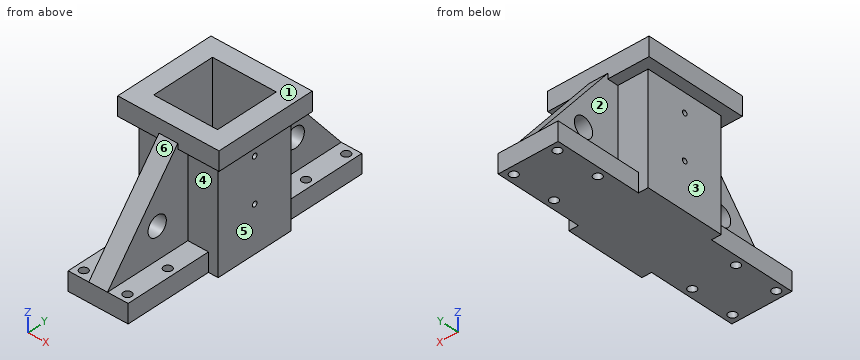
from build123d import *

# Parameters (mm, degrees)
SKETCH_W        = 48
SKETCH_H        = 15
PAD_DEPTH       = 203.2
SKETCH001_R     = 3.3
POCKET_DEPTH    = 15
SKETCH002_W     = 63.5
SKETCH002_H     = 63.5
PAD001_DEPTH    = 101.6
SKETCH003_W     = 51.05
SKETCH003_H     = 51.05
POCKET001_DEPTH = 88.9
SKETCH004_R     = 2
POCKET002_DEPTH = 15
SKETCH005_R     = 2
POCKET003_DEPTH = 15
PAD002_DEPTH    = 7.5
SKETCH007_W     = 81.05
SKETCH007_H     = 81.05
SKETCH007_W_2   = 51.05
SKETCH007_H_2   = 51.05
PAD003_DEPTH    = 15
SKETCH008_R     = 7.9375
POCKET004_DEPTH = 15


with BuildPart() as part:
    # Sketch → Pad (new body)
    with BuildSketch(Plane.XZ):
        with Locations((-24, 7.5)):
            Rectangle(SKETCH_W, SKETCH_H)
    extrude(amount=PAD_DEPTH)

    # Sketch001 (on Face4 of Pad) → Pocket (cut)
    with BuildSketch(Plane(origin=(0, 0, 0), x_dir=(1, 0, 0), z_dir=(0, 0, -1))):
        with Locations((-41.5, 41.5)):
            Circle(SKETCH001_R)
        with Locations((-6.5, 41.5)):
            Circle(SKETCH001_R)
        with Locations((-41.5, 6.5)):
            Circle(SKETCH001_R)
        with Locations((-6.5, 6.5)):
            Circle(SKETCH001_R)
        with Locations((-41.5, 196.7)):
            Circle(SKETCH001_R)
        with Locations((-6.5, 196.7)):
            Circle(SKETCH001_R)
        with Locations((-41.5, 161.7)):
            Circle(SKETCH001_R)
        with Locations((-6.5, 161.7)):
            Circle(SKETCH001_R)
    extrude(amount=-POCKET_DEPTH, mode=Mode.SUBTRACT)

    # Sketch002 (on Face2 of Pocket) → Pad001 (join)
    with BuildSketch(Plane(origin=(0, 0, 0), x_dir=(1, 0, 0), z_dir=(0, 0, -1))):
        with Locations((-24, 101.6)):
            Rectangle(SKETCH002_W, SKETCH002_H)
    extrude(amount=-PAD001_DEPTH)

    # Sketch003 (on Face11 of Pad001) → Pocket001 (cut)
    with BuildSketch(Plane(origin=(0, 0, 101.6), x_dir=(-1, 0, 0), z_dir=(0, 0, 1))):
        with Locations((24, 101.6)):
            Rectangle(SKETCH003_W, SKETCH003_H)
    extrude(amount=-POCKET001_DEPTH, mode=Mode.SUBTRACT)

    # Sketch004 (on Face11 of Pocket001) → Pocket002 (cut)
    with BuildSketch(Plane(origin=(7.75, 0, 0), x_dir=(0, 0, 1), z_dir=(1, 0, 0))):
        with Locations((71.6, 101.6)):
            Circle(SKETCH004_R)
        with Locations((36.6, 101.6)):
            Circle(SKETCH004_R)
    extrude(amount=-POCKET002_DEPTH, mode=Mode.SUBTRACT)

    # Sketch005 (on Face13 of Pocket002) → Pocket003 (cut)
    with BuildSketch(Plane(origin=(-55.75, 0, 0), x_dir=(0, 0, -1), z_dir=(-1, 0, 0))):
        with Locations((-71.6, 101.6)):
            Circle(SKETCH005_R)
        with Locations((-36.6, 101.6)):
            Circle(SKETCH005_R)
    extrude(amount=-POCKET003_DEPTH, mode=Mode.SUBTRACT)

    # Sketch006 (on Face11 of Pocket003) → Pad002 (join, symmetric)
    with BuildSketch(Plane(origin=(-24, 0, 0), x_dir=(0, 0, 1), z_dir=(1, 0, 0))):
        Polygon((15, 133.35), (15, 203.2), (101.6, 133.35), align=None)
        Polygon((101.6, 69.85), (15, 69.85), (15, 0), align=None)
    extrude(amount=PAD002_DEPTH, both=True)

    # Sketch007 (on Face13 of Pad002) → Pad003 (join)
    with BuildSketch(Plane(origin=(0, 0, 101.6), x_dir=(-1, 0, 0), z_dir=(0, 0, 1))):
        with Locations((24, 101.6)):
            Rectangle(SKETCH007_W, SKETCH007_H)
        with Locations((24, 101.6)):
            Rectangle(SKETCH007_W_2, SKETCH007_H_2, mode=Mode.SUBTRACT)
    extrude(amount=-PAD003_DEPTH)

    # Sketch008 (on Face34 of Pad003) → Pocket004 (cut)
    with BuildSketch(Plane(origin=(-16.5, 0, 0), x_dir=(0, 0, 1), z_dir=(1, 0, 0))):
        with Locations((40, 160)):
            Circle(SKETCH008_R)
        with Locations((40, 40)):
            Circle(SKETCH008_R)
    extrude(amount=-POCKET004_DEPTH, mode=Mode.SUBTRACT)


solid = part.part
Input: part model. Units: mm. Frame: model coordinates. Face numbers are marked on the shaded views. A direction names the side the tool comes from. Round coordinates to 2 decimals unless told otherwise and drop trailing zeros. Write each loop counter-clockwise with the first axis right and the second up, starting at its lowest first coordinate (ties: lowest second). Pieces come first, ordered by that corner, then holes.
1) Cut plane A-A (x = -6.5). Count the separate pieces of the cut face and the enclosed holes in it, then the cut area to 3 significant figures.
2) Cut plane C-C (y = -93.5). Return the cut outline in (x, z) (3 decimals).
3) Cut plane D-D (y = -16). Return the cut outline in (x, z).
4) Reachability of the marked faces 5 and 6 from +Z, -Z, +X, -X, +Y, -Y: full face, straight path, thin tool, end or side. Return the list, or none.
5) Draft query along Z for the marked faces 1, 2, 3 and 4. Return one class per face: pulls with the +Z half, pulls with the -Z half, needs draft (parallel to the pull), parting line crosses it, or undercut.
6) Cut plane B-B (z = 54). Return the cut outline in (x, y) (3 decimals), then the cut area to 3 significant figures.
7) Contact query for flat-ended pins moving along their axis: P1, Ø12, axis at y = -143.5, z = 12.5, coming from the +X side; P2, Ø8.5, axis at x = -6.5, y = -196.7, coming from the +Z side; P3, Ø21, axis at y = -180, z = 37.5, coming from the +X side. Output: stop coordinate, or through.
8) Ray query, L1, parallel to Y at x = -6.5, z = 12; L2, parallel to X at y = -41.5, z = 6.75; L3, parallel to Z at x = 4, y = -102. Return the intervals inside material, ascending.
Geometry says:
1. separate pieces: 5
1. enclosed holes: 0
1. area: 3,880 mm2
2. outline: (-64.525, 86.6) - (-55.75, 86.6) - (-55.75, 0) - (7.75, 0) - (7.75, 86.6) - (16.525, 86.6) - (16.525, 101.6) - (1.525, 101.6) - (1.525, 12.7) - (-49.525, 12.7) - (-49.525, 101.6) - (-64.525, 101.6) - close
3. outline: (-48, 0) - (0, 0) - (0, 15) - (-16.5, 15) - (-16.5, 34.84) - (-31.5, 34.84) - (-31.5, 15) - (-48, 15) - close
4. face 5: -Z, +X, +Y, -Y
4. face 6: +Z, +X, -X, -Y
5. face 1: pulls with the +Z half
5. face 2: undercut
5. face 3: needs draft
5. face 4: undercut
6. outline: (-55.75, -133.35) - (-31.5, -133.35) - (-31.5, -171.743) - (-16.5, -171.743) - (-16.5, -133.35) - (7.75, -133.35) - (7.75, -69.85) - (-16.5, -69.85) - (-16.5, -31.457) - (-31.5, -31.457) - (-31.5, -69.85) - (-55.75, -69.85) - close; hole (-49.525, -127.125) - (1.525, -127.125) - (1.525, -76.075) - (-49.525, -76.075) - close
6. area: 2,580 mm2
7. P1: stops at x = 0
7. P2: stops at z = 15
7. P3: stops at x = -16.5
8. L1: y = -203.2 to -200, -193.4 to -165, -158.4 to -44.8, -38.2 to -9.8, -3.2 to 0
8. L2: x = -48 to -44.8, -38.2 to -9.8, -3.2 to 0
8. L3: z = 0 to 34.64, 38.56 to 69.64, 73.56 to 101.6
